Design review of the part built by this model. Coordinates are the model's own, in mm. A direction names the side the tool comes from. Give positions to 0.01 mm unless a question says otherwise; leave off trailing zeros. Write each loop counter-clockwise with the first axis right and the second up, starting at its lowest first coordinate (ties: lowest second). Pieces come first, ordered by that corner, then holes.
```python
from build123d import *

# Parameters (mm, degrees)
F0_W     = 25
F0_H     = 25
F1_DEPTH = 3
F2_W     = 12.5
F2_H     = 12.5
F3_DEPTH = 1


with BuildPart() as f1:
    # F0 (on Top) → F1 (new body)
    with BuildSketch(Plane.XY):
        Rectangle(F0_W, F0_H)
    extrude(amount=F1_DEPTH)


with BuildPart() as f3:
    # F2 (on face) → F3 (new body)
    with BuildSketch(Plane.XY.offset(3)):
        Rectangle(F2_W, F2_H)
    extrude(amount=-F3_DEPTH)


with BuildPart() as f1_1:
    add(f1.part)

    # F4: cut F3
    add(f3.part, mode=Mode.SUBTRACT)


solid = f1_1.part
```
(1) Tool access review of faces 1 (the face through (6.25, -0.1, 2.5)), 2 (the face through (-12.5, 0, 1)): name each direction out of +Z, -Z, +X, -X, +Y, -Y from which nothing blocks a thin tool from reaching the whole face with its end or side.
Resolved:
face 1: +Z
face 2: +Z, -Z, -X, +Y, -Y
(2) Consider section A-A, the plane y = 4.75. Give the boundary of the cut face in (x, z), then the cut area to 3 significant figures.
Resolved:
outline: (-12.5, 0) - (12.5, 0) - (12.5, 3) - (6.25, 3) - (6.25, 2) - (-6.25, 2) - (-6.25, 3) - (-12.5, 3) - close
area: 62.5 mm2
(3) To check wall thickness, follow L1, parallel to X at y = -2, z = 2.7; L2, parallel to Z at x = 5, y = 0.75. State the ranges of each line that lie inside material, in increasing order.
Resolved:
L1: x = -12.5 to -6.25, 6.25 to 12.5
L2: z = 0 to 2
(4) Mouldability with a two-part tool opening along Y and no side actions: class faces 3 (the face through (0, -12.5, 1)), 4 (the face through (0, 0, 2)), 5 (the face through (0, 12.5, 1)), 6 (the face through (-9, 0, 3)) as pulls with the +Y half, pulls with the -Y half, needs draft (parallel to the pull), parting line crosses it, or undercut.
Resolved:
face 3: pulls with the -Y half
face 4: undercut
face 5: pulls with the +Y half
face 6: needs draft
